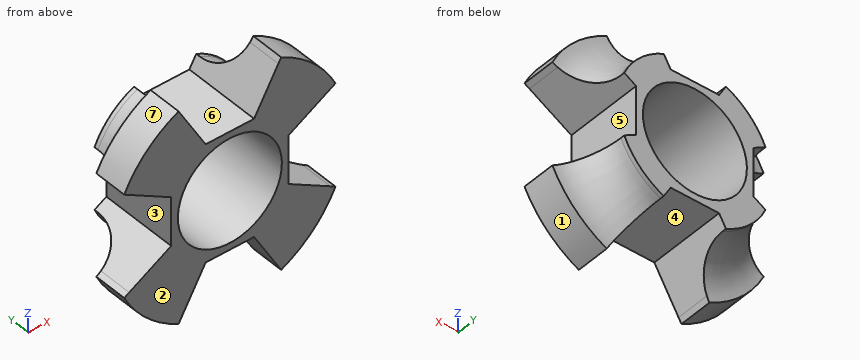
```python
from build123d import *

# Parameters (mm, degrees)
SKETCH1_R           = 11.5
SKETCH1_R_2         = 7.75
BOSS_EXTRUDE1_DEPTH = 11.4
SKETCH2_R           = 11.5
SKETCH2_R_2         = 7.75
BOSS_EXTRUDE2_DEPTH = 0.2
SKETCH5_R           = 17.5
SKETCH5_R_2         = 7.75
BOSS_EXTRUDE3_DEPTH = 5
FILLET1_R           = 6
CUT_EXTRUDE2_DEPTH  = 28.332398358
CIRPATTERN1_COUNT   = 4


with BuildPart() as part:
    # Sketch1 → Boss-Extrude1 (new body)
    with BuildSketch(Plane(origin=(0, 0, 0), x_dir=(1, 0, 0), z_dir=(0, 1, 0))):
        with Locations(Location((0, 0, 0), (0, 0, 270))):
            Circle(SKETCH1_R)
        with Locations(Location((0, 0, 0), (0, 0, 270))):
            Circle(SKETCH1_R_2, mode=Mode.SUBTRACT)
    extrude(amount=BOSS_EXTRUDE1_DEPTH)

    # Sketch2 → Boss-Extrude2 (add)
    with BuildSketch(Plane(origin=(0, 11.4, 0), x_dir=(1, 0, 0), z_dir=(0, 1, 0))):
        with Locations(Location((0, 0, 0), (0, 0, 270))):
            Circle(SKETCH2_R)
        with Locations(Location((0, 0, 0), (0, 0, 270))):
            Circle(SKETCH2_R_2, mode=Mode.SUBTRACT)
    extrude(amount=BOSS_EXTRUDE2_DEPTH)

    # Sketch5 → Boss-Extrude3 (add)
    with BuildSketch(Plane(origin=(0, 0, 0), x_dir=(1, 0, 0), z_dir=(0, 1, 0))):
        with Locations(Location((0, 0, 0), (0, 0, 270))):
            Circle(SKETCH5_R)
        with Locations(Location((0, 0, 0), (0, 0, 270))):
            Circle(SKETCH5_R_2, mode=Mode.SUBTRACT)
    extrude(amount=BOSS_EXTRUDE3_DEPTH)

    # Fillet1
    fillet1_edges = [part.edges().sort_by_distance(p)[0] for p in [
        (0, 5, -11.5),
    ]]
    fillet(fillet1_edges, radius=FILLET1_R - 0.0001)  # a hair under: the kernel refuses the full size

    # Sketch6 → Cut-Extrude2 (cut, through all)
    with BuildSketch(Plane(origin=(0, 11.6, 0), x_dir=(1, 0, 0), z_dir=(0, 1, 0))):
        Polygon((3.608439182, 21.25), (-3.608439182, 21.25), (-7.645118273, 15.741733278), (-7.216878365, 15), (-3.608439182, 8.75), (3.608439182, 8.75), (7.216878365, 15), (7.645118273, 15.741733278), align=None)
    cut_extrude2 = extrude(amount=-CUT_EXTRUDE2_DEPTH, mode=Mode.SUBTRACT)

    # CirPattern1: Cut-Extrude2 ×4 about axis
    cirpattern1_axis = Axis((0, 0, 0), (0, 1, 0))
    for i in range(1, CIRPATTERN1_COUNT):
        add(cut_extrude2.rotate(cirpattern1_axis, i * 360 / CIRPATTERN1_COUNT), mode=Mode.SUBTRACT)


solid = part.part
```
Source: CAD feature listing. Evaluate the final solid. Frame: model axes, mm. Face numbers are marked on the shaded views. A direction names the side the tool comes from. Round coordinates to 2 decimals unless told otherwise and drop trailing zeros. Loops run counter-clockwise (first coordinate to the right, second up) from the corner with the lowest first, then second, coordinate; pieces in that order, holes last.
1. Access query for the marked faces 4, 5, 6 and 7. Directions: +Z, -Z, +X, -X, +Y, -Y. A direction counts if a zero-diameter tool reaches every point of the face in a straight line with its end or side. Return the directions, or none.
2. Section query B-B on z = 0. Output: boundary loops of the cut face in (x, y).
3. Ray query, L1, parallel to X at y = 9.25, z = 0; L2, parallel to X at y = 6.25, z = -3; L3, parallel to Z at x = 12, y = 1.5. Return the intervals inside material, ascending.
4. Section query D-D on y = 6.5. Output: boundary loops of the cut face in (x, z).
5. Section query C-C on y = 1.25. Output: boundary loops of the cut face in (x, z).
6. Section query A-A on x = 0. Output: boundary loops of the cut face in (y, z).
7. Mould query, pull axis Z, two halves, no side actions, for the marked faces 1, 2 and 3. Classes: released by +Z, released by -Z, zero draft, split by the parting line, or undercut.
8. Contact query for flat-ended pins moving along their axis: pin 1 (6 mm diameter, centred on y = 6.5, z = -1, fed in from +X); pin 2 (2 mm diameter, centred on x = -0.5, y = 6, fed in from -Z); pin 3 (5 mm diameter, centred on y = 4.5, z = -10.5, fed in from -X). Output: stop coordinate, or through.
Answers below:
1. face 4: -Z, +Y, -Y
1. face 5: +X, +Y, -Y
1. face 6: +Z, +Y, -Y
1. face 7: +Z, -X, +Y, -Y
2. outline: (-8.75, 0) - (-7.75, 0) - (-7.75, 11.6) - (-8.75, 11.6) - close; (7.75, 0) - (8.75, 0) - (8.75, 11.6) - (7.75, 11.6) - close
3. L1: x = -8.75 to -7.75, 7.75 to 8.75
3. L2: x = -8.75 to -7.15, 7.15 to 8.75
3. L3: z = -12.74 to -5.48, 5.48 to 12.74
4. outline: (-12.29, -5.65) arc R13.53 ccw to (-5.65, -12.29) - (-3.61, -8.75) - (3.61, -8.75) - (5.65, -12.29) arc R13.53 ccw to (12.29, -5.65) - (8.75, -3.61) - (8.75, 3.61) - (12.29, 5.65) arc R13.53 ccw to (5.65, 12.29) - (3.61, 8.75) - (-3.61, 8.75) - (-5.65, 12.29) arc R13.53 ccw to (-12.29, 5.65) - (-8.75, 3.61) - (-8.75, -3.61) - close; hole circle Ø15.5 at (0, 0)
5. outline: (-15.74, -7.65) arc R17.5 ccw to (-7.65, -15.74) - (-3.61, -8.75) - (3.61, -8.75) - (7.65, -15.74) arc R17.5 ccw to (15.74, -7.65) - (8.75, -3.61) - (8.75, 3.61) - (15.74, 7.65) arc R17.5 ccw to (7.65, 15.74) - (3.61, 8.75) - (-3.61, 8.75) - (-7.65, 15.74) arc R17.5 ccw to (-15.74, 7.65) - (-8.75, 3.61) - (-8.75, -3.61) - close; hole circle Ø15.5 at (0, 0)
6. outline: (0, -8.75) - (11.6, -8.75) - (11.6, -7.75) - (0, -7.75) - close; (0, 7.75) - (11.6, 7.75) - (11.6, 8.75) - (0, 8.75) - close
7. face 1: released by -Z
7. face 2: zero draft
7. face 3: undercut
8. pin 1: stops at x = 9.43
8. pin 2: stops at z = -8.75
8. pin 3: stops at x = -15.56
